Part model, mm, in its own coordinate system. Face numbers are marked on the shaded views. A direction names the side the tool comes from. Give positions to 0.01 mm unless a question says otherwise; leave off trailing zeros. Order: outer loops, then holes, each group sorted by start corner. A loop starts at its lowest first (then second) coordinate and runs counter-clockwise, first axis right, second up.
from build123d import *

# Parameters (mm, degrees)
PROFIL_BASE_R                = 75
BASE_DEPTH                   = 50
BASE_TAPER                   = 25
CONG_1_R                     = 10
PIED_DEPTH                   = 50
R_P_TITION_CIRCULAIRE1_COUNT = 5
ESQUISSE3_R                  = 45.313914484
BOSS_EXTRU_3_DEPTH           = 50
BOSS_EXTRU_3_TAPER           = 40
ESQUISSE5_R                  = 1
BOSS_EXTRU_4_DEPTH           = 50
CONG_2_R                     = 1
CHANFREIN1_SIZE              = 0.254371318
CHANFREIN1_SIZE_2            = 11
CONG_3_R                     = 1
CONG_4_R                     = 1


with BuildPart() as part:
    # profil Base → Base (new body)
    with BuildSketch(Plane(origin=(0, 0, 0), x_dir=(1, 0, 0), z_dir=(0, 1, 0))):
        Circle(PROFIL_BASE_R)
    extrude(amount=BASE_DEPTH, taper=BASE_TAPER)

    # Congé1
    cong_1_edges = [part.edges().sort_by_distance(p)[0] for p in [
        (-51.684617092, 50, 0),
    ]]
    fillet(cong_1_edges, radius=CONG_1_R)

    # Profil Pied → Pied (add)
    with BuildSketch(Plane.XZ):
        with BuildLine():
            Line((-75, 0), (-45, 0))
            ThreePointArc((-45, 0), (-43.93332032, 9.739782627), (-40.783850417, 19.017821778))
            Line((-40.783850417, 19.017821778), (-67.973084028, 31.696369631))
            ThreePointArc((-67.973084028, 31.696369631), (-73.222200534, 16.232971045), (-75, 0))
        make_face()
    pied = extrude(amount=PIED_DEPTH)

    # Répétition circulaire1: Pied ×5 about axis
    r_p_tition_circulaire1_axis = Axis((0, 0, 0), (0, 1, 0))
    for i in range(1, R_P_TITION_CIRCULAIRE1_COUNT):
        add(pied.rotate(r_p_tition_circulaire1_axis, i * 360 / R_P_TITION_CIRCULAIRE1_COUNT))

    # Esquisse3 → Boss.-Extru.3 (add)
    with BuildSketch(Plane(origin=(0, 50, 0), x_dir=(1, 0, 0), z_dir=(0, 1, 0))):
        Circle(ESQUISSE3_R)
    extrude(amount=BOSS_EXTRU_3_DEPTH, taper=BOSS_EXTRU_3_TAPER)

    # Esquisse5 → Boss.-Extru.4 (add)
    with BuildSketch(Plane(origin=(0, 100, 0), x_dir=(1, 0, 0), z_dir=(0, 1, 0))):
        with Locations(Location((0, 0, 0), (0, 0, 270))):
            Circle(ESQUISSE5_R)
    extrude(amount=BOSS_EXTRU_4_DEPTH)

    # Congé2
    cong_2_edges = [part.edges().sort_by_distance(p)[0] for p in [
        (0, 150, -1),
    ]]
    fillet(cong_2_edges, radius=CONG_2_R)

    # Chanfrein1
    # the kernel refuses this chamfer: 11, 0.254371318 mm, written as the material it takes off along each edge
    with BuildSketch(Plane(origin=(0, 100, 0), x_dir=(1, 0, 0), z_dir=(0, 0, -1))) as chanfrein1_piece_1:
        Polygon((3.358932925 - CHANFREIN1_SIZE, 0), (3.358932925 + CHANFREIN1_SIZE_2 * 0.642787609687, CHANFREIN1_SIZE_2 * 0.766044443119), (3.358932925, 0), align=None)
    revolve(axis=Axis((0, 100, 0), (0, -1, 0)), mode=Mode.SUBTRACT)

    # Congé3
    cong_3_edges = [part.edges().sort_by_distance(p)[0] for p in [
        (-3.104561607, 100, 0),
    ]]
    fillet(cong_3_edges, radius=CONG_3_R)

    # Congé4
    cong_4_edges = [part.edges().sort_by_distance(p)[0] for p in [
        (0, 100, -1),
    ]]
    fillet(cong_4_edges, radius=CONG_4_R)


solid = part.part
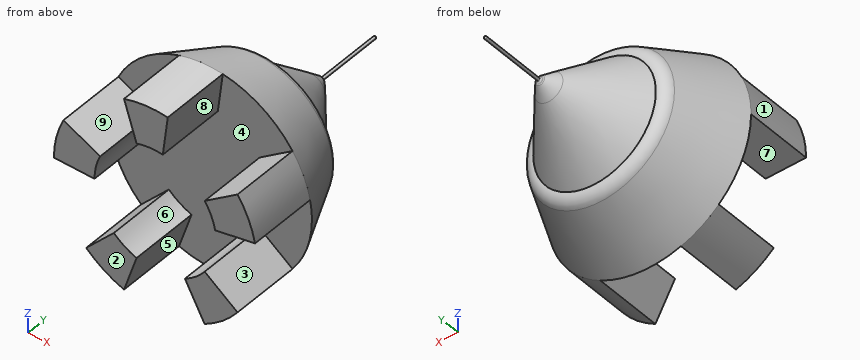
Item 1: Drop flat-ended pins along their axis: P1, Ø1.5, axis at x = 27.5, z = -4.5, coming from the +Y side; P2, Ø4, axis at y = 57, z = 3.5, coming from the -X side; P3, Ø12, axis at y = 23.5, z = 8.5, coming from the +X side. Give the stop position or say it passes through.
Item 2: Band-saw the part on B-B on y = 73. List the corners of the cut face in (x, z), plus the area to 3 significant figures.
Item 3: Band-saw the part on A-A on y = 128.5. List the corners of the cut face in (x, z).
Item 4: Pull direction Z, two halves, no side cores. Call the marked faces 1, 2, 3 and 4: released by +Z, released by -Z, zero draft, split by the parting line, or undercut.
Item 5: Which spindle directions (+Z, -Z, +X, -X, +Y, -Y) get a long thin tool onto all of the face, cutting with end or side? Do the marked faces 5, 6, 7, 8 and 9. Say none if no direction does.
Item 6: Drill centre lines: probe 1 along X at (y, z) = (-1.5, -49); probe 2 along Y at (x, z) = (34, 30.5); probe 3 along X at (y, z) = (-11.5, 16). Where is each one in solid material? Low to high.
Working result:
1. P1: stops at y = 71.69
1. P2: stops at x = -40.98
1. P3: stops at x = 66.38
2. outline: circle Ø52.03 at (0, 0)
2. area: 2,130 mm2
3. outline: circle Ø2 at (0, 0)
4. face 1: released by +Z
4. face 2: zero draft
4. face 3: undercut
4. face 4: undercut
5. face 5: -Z, -Y
5. face 6: -Y
5. face 7: +X, -X, -Y
5. face 8: -Z, +X, -Y
5. face 9: +Z, -Y
6. probe 1: x = -45.69 to -15.92, 27.16 to 56.78
6. probe 2: y = 0 to 49.99
6. probe 3: x = -73.27 to -42.06, 42.06 to 73.27
